from build123d import *

# Parameters (mm, degrees)
GE_22344_OUTLINE_R = 5.357876
GE_22344_DEPTH     = 6.35
CUT_EXTRUDE1_START = -5.842
CUT_EXTRUDE1_DEPTH = 5.842


# Read off the part's stored shape, not the designer's step: GE-22344
with BuildPart() as part:
    # GE-22344 outline → GE-22344 (new body)
    with BuildSketch(Plane.XY):
        with BuildLine():
            Line((7.3025, 0), (583.2475, 0))
            ThreePointArc((583.2475, 0), (585.043551224, 0.743948776), (585.7875, 2.54))
            Line((585.7875, 2.54), (585.7875, 568.96))
            ThreePointArc((585.7875, 568.96), (585.043551224, 570.756051224), (583.2475, 571.5))
            Line((583.2475, 571.5), (501.015, 571.5))
            ThreePointArc((501.015, 571.5), (499.218948776, 570.756051224), (498.475, 568.96))
            Line((498.475, 568.96), (498.475, 508))
            ThreePointArc((498.475, 508), (494.755256121, 499.019743879), (485.775, 495.3))
            Line((485.775, 495.3), (466.725, 495.3))
            ThreePointArc((466.725, 495.3), (457.744743879, 499.019743879), (454.025, 508))
            Line((454.025, 508), (454.025, 568.96))
            ThreePointArc((454.025, 568.96), (453.281051224, 570.756051224), (451.485, 571.5))
            Line((451.485, 571.5), (24.765, 571.5))
            ThreePointArc((24.765, 571.5), (22.968948776, 570.756051224), (22.225, 568.96))
            Line((22.225, 568.96), (22.225, 508))
            ThreePointArc((22.225, 508), (18.505256121, 499.019743879), (9.525, 495.3))
            Line((9.525, 495.3), (-9.525, 495.3))
            ThreePointArc((-9.525, 495.3), (-18.505256121, 499.019743879), (-22.225, 508))
            Line((-22.225, 508), (-22.225, 568.96))
            ThreePointArc((-22.225, 568.96), (-22.968948776, 570.756051224), (-24.765, 571.5))
            Line((-24.765, 571.5), (-451.485, 571.5))
            ThreePointArc((-451.485, 571.5), (-453.281051224, 570.756051224), (-454.025, 568.96))
            Line((-454.025, 568.96), (-454.025, 508))
            ThreePointArc((-454.025, 508), (-457.744743879, 499.019743879), (-466.725, 495.3))
            Line((-466.725, 495.3), (-485.775, 495.3))
            ThreePointArc((-485.775, 495.3), (-494.755256121, 499.019743879), (-498.475, 508))
            Line((-498.475, 508), (-498.475, 568.96))
            ThreePointArc((-498.475, 568.96), (-499.218948776, 570.756051224), (-501.015, 571.5))
            Line((-501.015, 571.5), (-583.2475, 571.5))
            ThreePointArc((-583.2475, 571.5), (-585.043551224, 570.756051224), (-585.7875, 568.96))
            Line((-585.7875, 568.96), (-585.7875, 2.54))
            ThreePointArc((-585.7875, 2.54), (-585.043551224, 0.743948776), (-583.2475, 0))
            Line((-583.2475, 0), (-7.3025, 0))
            ThreePointArc((-7.3025, 0), (-5.506448776, 0.743948776), (-4.7625, 2.54))
            Line((-4.7625, 2.54), (-4.7625, 11.1125))
            ThreePointArc((-4.7625, 11.1125), (0, 15.875), (4.7625, 11.1125))
            Line((4.7625, 11.1125), (4.7625, 2.54))
            ThreePointArc((4.7625, 2.54), (5.506448776, 0.743948776), (7.3025, 0))
        make_face()
        with Locations((-304.8, 76.2)):
            Circle(GE_22344_OUTLINE_R, mode=Mode.SUBTRACT)
        with Locations((-247.65, 76.2)):
            Circle(GE_22344_OUTLINE_R, mode=Mode.SUBTRACT)
        with Locations((247.65, 76.2)):
            Circle(GE_22344_OUTLINE_R, mode=Mode.SUBTRACT)
        with Locations((304.8, 76.2)):
            Circle(GE_22344_OUTLINE_R, mode=Mode.SUBTRACT)
        with Locations((-304.8, 495.3)):
            Circle(GE_22344_OUTLINE_R, mode=Mode.SUBTRACT)
        with Locations((-247.65, 495.3)):
            Circle(GE_22344_OUTLINE_R, mode=Mode.SUBTRACT)
        with Locations((247.65, 495.3)):
            Circle(GE_22344_OUTLINE_R, mode=Mode.SUBTRACT)
        with Locations((304.8, 495.3)):
            Circle(GE_22344_OUTLINE_R, mode=Mode.SUBTRACT)
    extrude(amount=GE_22344_DEPTH)

    # Sketch4 → Cut-Extrude1 (cut)
    with BuildSketch(Plane.XY.offset(6.35).offset(CUT_EXTRUDE1_START)):
        with BuildLine():
            Line((-583.2475, 0), (-7.3025, 0))
            ThreePointArc((-7.3025, 0), (-5.506448776, 0.743948776), (-4.7625, 2.54))
            Line((-4.7625, 2.54), (-4.7625, 11.1125))
            ThreePointArc((-4.7625, 11.1125), (0, 15.875), (4.7625, 11.1125))
            Line((4.7625, 11.1125), (4.7625, 2.54))
            ThreePointArc((4.7625, 2.54), (5.506448776, 0.743948776), (7.3025, 0))
            Line((7.3025, 0), (583.2475, 0))
            ThreePointArc((583.2475, 0), (585.043551224, 0.743948776), (585.7875, 2.54))
            Line((585.7875, 2.54), (585.7875, 568.96))
            ThreePointArc((585.7875, 568.96), (585.043551224, 570.756051224), (583.2475, 571.5))
            Line((583.2475, 571.5), (501.015, 571.5))
            ThreePointArc((501.015, 571.5), (499.218948776, 570.756051224), (498.475, 568.96))
            Line((498.475, 568.96), (498.475, 508))
            ThreePointArc((498.475, 508), (494.755256121, 499.019743879), (485.775, 495.3))
            Line((485.775, 495.3), (466.725, 495.3))
            ThreePointArc((466.725, 495.3), (457.744743879, 499.019743879), (454.025, 508))
            Line((454.025, 508), (454.025, 568.96))
            ThreePointArc((454.025, 568.96), (453.281051224, 570.756051224), (451.485, 571.5))
            Line((451.485, 571.5), (24.765, 571.5))
            ThreePointArc((24.765, 571.5), (22.968948776, 570.756051224), (22.225, 568.96))
            Line((22.225, 568.96), (22.225, 508))
            ThreePointArc((22.225, 508), (18.505256121, 499.019743879), (9.525, 495.3))
            Line((9.525, 495.3), (-9.525, 495.3))
            ThreePointArc((-9.525, 495.3), (-18.505256121, 499.019743879), (-22.225, 508))
            Line((-22.225, 508), (-22.225, 568.96))
            ThreePointArc((-22.225, 568.96), (-22.968948776, 570.756051224), (-24.765, 571.5))
            Line((-24.765, 571.5), (-451.485, 571.5))
            ThreePointArc((-451.485, 571.5), (-453.281051224, 570.756051224), (-454.025, 568.96))
            Line((-454.025, 568.96), (-454.025, 508))
            ThreePointArc((-454.025, 508), (-457.744743879, 499.019743879), (-466.725, 495.3))
            Line((-466.725, 495.3), (-485.775, 495.3))
            ThreePointArc((-485.775, 495.3), (-494.755256121, 499.019743879), (-498.475, 508))
            Line((-498.475, 508), (-498.475, 568.96))
            ThreePointArc((-498.475, 568.96), (-499.218948776, 570.756051224), (-501.015, 571.5))
            Line((-501.015, 571.5), (-583.2475, 571.5))
            ThreePointArc((-583.2475, 571.5), (-585.043551224, 570.756051224), (-585.7875, 568.96))
            Line((-585.7875, 568.96), (-585.7875, 2.54))
            ThreePointArc((-585.7875, 2.54), (-585.043551224, 0.743948776), (-583.2475, 0))
        make_face()
    extrude(amount=CUT_EXTRUDE1_DEPTH, mode=Mode.SUBTRACT)


solid = part.part
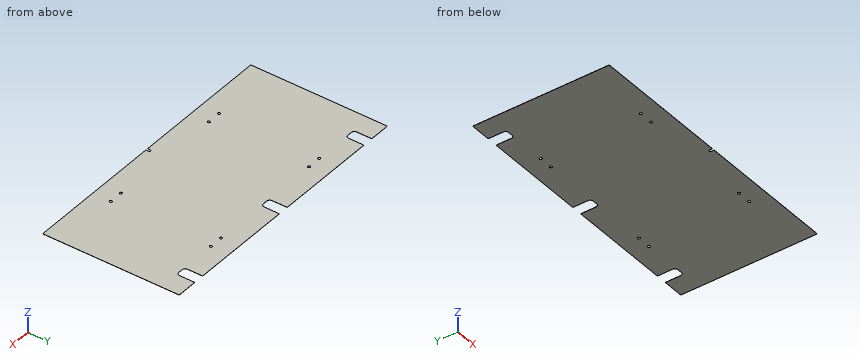
Part model, mm, in its own coordinate system. Give positions to 0.01 mm unless a question says otherwise; leave off trailing zeros. Put each result on its own line as item: value. Start each with the question number.
1) Flat gauge pins, fed straight in: pin 1 (9.5 mm diameter, centred on x = 247.65, y = 495.3, fed in from +Z); pin 2 (12.5 mm diameter, centred on x = -304.8, y = 76.2, fed in from +Z). Where does each tip first touch, or does it go through?
2) Probe probe 1 along X at (y, z) = (76.2, 0.4); probe 2 along Y at (x, z) = (-304.8, 0.15); probe 3 along Y at (x, z) = (19, 0.25). List the from-to ranges inside material, lowest first.
3) Saw through at A-A (z = 0.2). State how many separate pieces and enclosed holes the cut face has, then the cut area to 3 significant figures.
Numbers:
1. pin 1: through
1. pin 2: z = 0.51
2. probe 1: -585.79 to -310.16, -299.44 to -253.01, -242.29 to 242.29, 253.01 to 299.44, 310.16 to 585.79
2. probe 2: 0 to 70.84, 81.56 to 489.94, 500.66 to 571.5
2. probe 3: 0 to 499.54
3. separate pieces: 1
3. enclosed holes: 8
3. area: 659,000 mm^2
